Verification items for this drawing (mm, ordinates from the low corner). Coordinates: 2 decimals unless noted, no trailing zeros. Loops run counter-clockwise (first coordinate to the right, second up) from the corner with the lowest first, then second, coordinate; pieces in that order, holes last. Notation, with made-up numbers: M 75.25,69 L 93.25,69 A24 cw 93.25,87 Z; hole C 15.5,-0.5 d6. An arc over 180 degrees is marked long. Use CSV: the item, a comma, the result in double quotes.
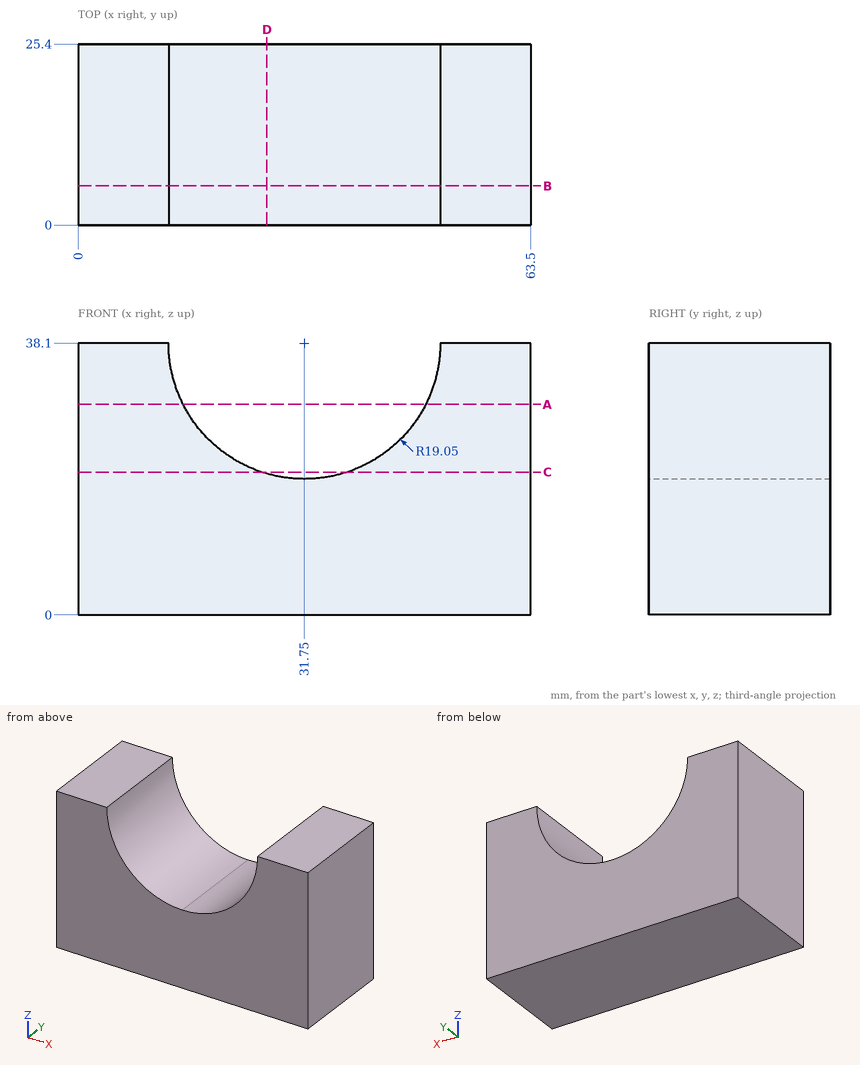
1. Thickness scan on line 1 (X direction, y = 19.25, z = 23.5); line 2 (X direction, y = 16.5, z = 21.5); line 3 (Z direction, x = 41.5, y = 10.75). Record the ranges inside material, lowest first. Write a range as [from, to].
The answers:
line 1,"[0, 19.51], [43.99, 63.5]"
line 2,"[0, 22.4], [41.1, 63.5]"
line 3,"[0, 21.73]"
2. Section check B-B, the plane y = 5.5. Record the cut outline in (x, z), plus the area to 3 significant figures.
The answers:
outline,"M 0,0 L 63.5,0 L 63.5,38.1 L 50.8,38.1 A19.05 cw 31.75,19.05 A19.05 cw 12.7,38.1 L 0,38.1 Z"
area,"1,850 mm^2"
3. Section check A-A, the plane z = 29.5. Record the cut outline in (x, y).
The answers:
outline,"M 0,0 L 14.75,0 L 14.75,25.4 L 0,25.4 Z; M 48.75,0 L 63.5,0 L 63.5,25.4 L 48.75,25.4 Z"
4. Section check D-D, the plane x = 26.5. Record the cut outline in (y, z).
The answers:
outline,"M 0,0 L 25.4,0 L 25.4,19.79 L 0,19.79 Z"
5. Section check C-C, the plane z = 20. Record the cut outline in (x, y).
The answers:
outline,"M 0,0 L 25.81,0 L 25.81,25.4 L 0,25.4 Z; M 37.69,0 L 63.5,0 L 63.5,25.4 L 37.69,25.4 Z"
6. Gauge pin test, flat end, axial feed: P1, Ø5, axis at x = 40.5, y = 21.5, coming from the +Z side. Record the tip position at first contact, or that the pin passes through.
The answers:
P1,"z = 22.73"
